```python
from build123d import *

# Parameters (mm, degrees)
SKETCH2_W           = 30.48
SKETCH2_H           = 38.1
SKETCH2_R           = 2.159
BOSS_EXTRUDE1_DEPTH = 4.826
SKETCH3_W           = 30.48
SKETCH3_H           = 4.826
BOSS_EXTRUDE2_DEPTH = 74.676
SKETCH4_W           = 4.826
SKETCH4_H           = 30.48
BOSS_EXTRUDE4_DEPTH = 33.274
SKETCH5_W           = 50.8
SKETCH5_H           = 6.35
BOSS_EXTRUDE5_DEPTH = 12.7
CUT_EXTRUDE1_REACH  = 14.7
SKETCH6_R           = 1.6
FILLET2_R           = 4
SKETCH7_R           = 4.5
BOSS_EXTRUDE6_DEPTH = 6.35


with BuildPart() as part:
    # Sketch2 → Boss-Extrude1 (new body)
    with BuildSketch(Plane(origin=(0, 0, 0), x_dir=(0, 0, -1), z_dir=(1, 0, 0))):
        with Locations((15.24, 19.05)):
            Rectangle(SKETCH2_W, SKETCH2_H)
        with Locations((5.715, 6.05)):
            Circle(SKETCH2_R, mode=Mode.SUBTRACT)
        with Locations((24.765, 6.05)):
            Circle(SKETCH2_R, mode=Mode.SUBTRACT)
    extrude(amount=BOSS_EXTRUDE1_DEPTH)

    # Sketch3 → Boss-Extrude2 (add)
    with BuildSketch(Plane.ZY):
        with Locations((-15.24, 35.687)):
            Rectangle(SKETCH3_W, SKETCH3_H)
    extrude(amount=BOSS_EXTRUDE2_DEPTH)

    # Sketch4 → Boss-Extrude4 (add)
    with BuildSketch(Plane.XZ.offset(-33.274)):
        with Locations((-72.263, -15.24)):
            Rectangle(SKETCH4_W, SKETCH4_H)
    extrude(amount=BOSS_EXTRUDE4_DEPTH)

    # Sketch5 → Boss-Extrude5 (add)
    with BuildSketch(Plane(origin=(0, 38.1, 0), x_dir=(1, 0, 0), z_dir=(0, 1, 0))):
        with Locations((-34.925, 9.525)):
            Rectangle(SKETCH5_W, SKETCH5_H)
    extrude(amount=BOSS_EXTRUDE5_DEPTH)

    # Sketch6 → Cut-Extrude1 (cut, up to next)
    with BuildSketch(Plane(origin=(0, 0, -12.7), x_dir=(-1, 0, 0), z_dir=(0, 0, -1)), mode=Mode.PRIVATE) as cut_extrude1_sk1:
        with Locations((16.425, 44.5)):
            Circle(SKETCH6_R)
    cut_extrude1_tool1 = extrude(cut_extrude1_sk1.sketch, amount=-CUT_EXTRUDE1_REACH, mode=Mode.PRIVATE) & part.part
    add(cut_extrude1_tool1.solids().sort_by_distance((-16.425, 44.5, -12.7))[0], mode=Mode.SUBTRACT)
    # Sketch6 → Cut-Extrude1 (cut, up to next)
    with BuildSketch(Plane(origin=(0, 0, -12.7), x_dir=(-1, 0, 0), z_dir=(0, 0, -1)), mode=Mode.PRIVATE) as cut_extrude1_sk2:
        with Locations((53.425, 44.5)):
            Circle(SKETCH6_R)
    cut_extrude1_tool2 = extrude(cut_extrude1_sk2.sketch, amount=-CUT_EXTRUDE1_REACH, mode=Mode.PRIVATE) & part.part
    add(cut_extrude1_tool2.solids().sort_by_distance((-53.425, 44.5, -12.7))[0], mode=Mode.SUBTRACT)

    # Fillet2
    fillet2_edges = [part.edges().sort_by_distance(p)[0] for p in [
        (4.826, 38.1, -15.24),
        (-74.676, 38.1, -15.24),
        (-60.325, 38.1, -9.525),
        (-9.525, 38.1, -9.525),
        (-60.325, 50.8, -9.525),
        (-9.525, 50.8, -9.525),
    ]]
    fillet(fillet2_edges, radius=FILLET2_R)

    # Sketch7 → Boss-Extrude6 (add)
    with BuildSketch(Plane(origin=(-69.85, 0, 0), x_dir=(0, 0, -1), z_dir=(1, 0, 0))):
        with Locations((15.24, 6.096)):
            Circle(SKETCH7_R)
    extrude(amount=BOSS_EXTRUDE6_DEPTH)


solid = part.part
```
Design review of the part built by this model. Coordinates are the model's own, in mm. A direction names the side the tool comes from. Coordinates: 2 decimals unless noted, no trailing zeros. Order: outer loops, then holes, each group sorted by start corner. A loop starts at its lowest first (then second) coordinate and runs counter-clockwise, first axis right, second up. Notation, with made-up numbers: (-27.75, 52.25) - (-14.75, 52.25) arc R24 cw to (-14.75, 64.25) - close; hole circle Ø10 at (-33, 15). An arc over 180 degrees is marked (long way). One line per question, with ' | ' between items.
Q1. For faces 1 (the flat face through (-60.325, 44, -9)), 2 (the cylindrical face through (2.38, 3.94, -5.25)), 3 (the flat face through (0, 17, -15)), 4 (the flat face through (-35, 44, -6.35)), list the 3-axis set-ups (+Z, -Z, +X, -X, +Y, -Y) from which the entire face can be reached by the end or side of a thin tool; tool diameter is ignored.
Answer key:
face 1: +Z, -Z, -X, +Y | face 2: +X | face 3: +Z, -Z, -Y | face 4: +Z, +X, -X, +Y
Q2. Consider section B-B, the plane y = 28.5. Give the boundary of the cut face in (x, z), then the cut area to 3 significant figures.
Answer key:
outline: (-74.68, -30.48) - (-69.85, -30.48) - (-69.85, 0) - (-74.68, 0) - close; (0, -30.48) - (4.83, -30.48) - (4.83, 0) - (0, 0) - close | area: 294 mm2
Q3. Consider section C-C, the plane x = -25. Give the boundary of the cut face in (y, z), then the cut area to 3 significant figures.
Answer key:
outline: (33.27, -30.48) - (38.1, -30.48) - (38.1, -12.7) - (50.8, -12.7) - (50.8, -6.35) - (38.1, -6.35) - (38.1, 0) - (33.27, 0) - close | area: 228 mm2
Q4. Consider section A-A, the plane y = 44.5. Give the boundary of the cut face in (x, z) (3 decimals).
Answer key:
outline: (-60.325, -12.7) - (-55.025, -12.7) - (-55.025, -6.35) - (-60.325, -6.35) - close; (-51.825, -12.7) - (-18.025, -12.7) - (-18.025, -6.35) - (-51.825, -6.35) - close; (-14.825, -12.7) - (-9.525, -12.7) - (-9.525, -6.35) - (-14.825, -6.35) - close
Q5. To check wall thickness, follow line 1 along Z through (x, y) = (2, 6); line 2 along X through (y, z) = (29.5, -29). State the ranges of each line that lie inside material, in increasing order.
Answer key:
line 1: z = -30.48 to -26.92, -22.61 to -7.87, -3.56 to 0 | line 2: x = -74.68 to -69.85, 0 to 4.83
Q6. Consider section D-D, the plane z = -15.24. Give the boundary of the cut face in (x, y).
Answer key:
outline: (-74.68, 0) - (-69.85, 0) - (-69.85, 1.6) - (-63.5, 1.6) - (-63.5, 10.6) - (-69.85, 10.6) - (-69.85, 33.27) - (0, 33.27) - (0, 0) - (4.83, 0) - (4.83, 34.1) arc R4 ccw to (0.83, 38.1) - (-70.68, 38.1) arc R4 ccw to (-74.68, 34.1) - close
Q7. The part is to be moulded in two halves that separate along X. For faces 5 (the cylindrical face through (3.62, 36.96, -15.45)), 6 (the flat face through (-35, 35, -30.48)), 7 (the flat face through (-63.5, 6, -15)), say which applies: +X half, -X half, draft (parallel to the pull), parting line (faces both ways), or undercut.
Answer key:
face 5: +X half | face 6: draft | face 7: undercut
Q8. Clearance check with flat-ended pins moving along their axes: pin 1 Ø1 at (x, z) = (-6, -6.5) entering from +Y; pin 2 Ø1.4 at (y, z) = (45.5, -9.5) entering from -X (3 decimals); pin 3 Ø10 at (x, y) = (-35, 46.5) entering from +Z. State where each tip first meets the part, or that it passes through.
Answer key:
pin 1: stops at y = 38.22 | pin 2: stops at x = -60.325 | pin 3: stops at z = -6.35
